from build123d import *

# Parameters (mm, degrees)
SKETCH1_W            = 182
SKETCH1_H            = 33.5
BOSS_EXTRUDE1_DEPTH  = 1.6
SKETCH2_R            = 1.75
CUT_EXTRUDE1_DEPTH   = 1.6
LPATTERN1_COUNT      = 2
LPATTERN1_PITCH      = 175
LPATTERN1_COUNT_DIR2 = 2
LPATTERN1_PITCH_DIR2 = 26.5
SKETCH3_W            = 161.4
SKETCH3_H            = 28.9
BOSS_EXTRUDE2_DEPTH  = 8.95
SKETCH3_2_W          = 161.4
SKETCH3_2_H          = 28.9
BOSS_EXTRUDE3_DEPTH  = 4.65
SKETCH4_W            = 154.4
SKETCH4_H            = 16.5
CUT_EXTRUDE2_DEPTH   = 1
FILLET1_R            = 1
FILLET2_R            = 1
FILLET3_R            = 1
FILLET4_R            = 1


with BuildPart() as part:
    # Sketch1 → Boss-Extrude1 (new body)
    with BuildSketch(Plane(origin=(0, 0, 0), x_dir=(1, 0, 0), z_dir=(0, 1, 0))):
        with Locations((10.727604206, -13.815258398)):
            Rectangle(SKETCH1_W, SKETCH1_H)
    extrude(amount=BOSS_EXTRUDE1_DEPTH)

    # Sketch2 → Cut-Extrude1 (cut)
    with BuildSketch(Plane(origin=(0, 1.6, 0), x_dir=(1, 0, 0), z_dir=(0, 1, 0))):
        with Locations(Location((-76.772395794, -0.565258398, 0), (0, 0, 270))):
            Circle(SKETCH2_R)
    cut_extrude1 = extrude(amount=-CUT_EXTRUDE1_DEPTH, mode=Mode.SUBTRACT)

    # LPattern1: Cut-Extrude1 2 × 2
    with Locations(*[(i * LPATTERN1_PITCH, 0, j * LPATTERN1_PITCH_DIR2) for i in range(LPATTERN1_COUNT) for j in range(LPATTERN1_COUNT_DIR2) if (i, j) != (0, 0)]):
        add(cut_extrude1, mode=Mode.SUBTRACT)

    # Sketch3 → Boss-Extrude2 (add)
    with BuildSketch(Plane(origin=(0, 1.6, 0), x_dir=(1, 0, 0), z_dir=(0, 1, 0))):
        with Locations((13.227604206, -13.815258398)):
            Rectangle(SKETCH3_W, SKETCH3_H)
    extrude(amount=BOSS_EXTRUDE2_DEPTH)

    # Sketch3_2 → Boss-Extrude3 (add)
    with BuildSketch(Plane(origin=(0, 1.6, 0), x_dir=(1, 0, 0), z_dir=(0, 1, 0))):
        with Locations((13.227604206, -13.815258398)):
            Rectangle(SKETCH3_2_W, SKETCH3_2_H)
    extrude(amount=-BOSS_EXTRUDE3_DEPTH)

    # Sketch4 → Cut-Extrude2 (cut)
    with BuildSketch(Plane(origin=(0, 10.55, 0), x_dir=(1, 0, 0), z_dir=(0, 1, 0))):
        with Locations((13.227604206, -13.815258398)):
            Rectangle(SKETCH4_W, SKETCH4_H)
    extrude(amount=-CUT_EXTRUDE2_DEPTH, mode=Mode.SUBTRACT)

    # Fillet1
    fillet1_edges = [part.edges().sort_by_distance(p)[0] for p in [
        (-63.972395794, 10.05, 5.565258398),
    ]]
    fillet(fillet1_edges, radius=FILLET1_R)

    # Fillet2
    fillet2_edges = [part.edges().sort_by_distance(p)[0] for p in [
        (-63.972395794, 10.05, 22.065258398),
    ]]
    fillet(fillet2_edges, radius=FILLET2_R)

    # Fillet3
    fillet3_edges = [part.edges().sort_by_distance(p)[0] for p in [
        (90.427604206, 10.05, 5.565258398),
    ]]
    fillet(fillet3_edges, radius=FILLET3_R)

    # Fillet4
    fillet4_edges = [part.edges().sort_by_distance(p)[0] for p in [
        (90.427604206, 10.05, 22.065258398),
    ]]
    fillet(fillet4_edges, radius=FILLET4_R)


solid = part.part
Could you check a few things on this model? Use its own coordinates, in mm. A direction names the side the tool comes from. Coordinates: 2 decimals unless noted, no trailing zeros. Loops run counter-clockwise (first coordinate to the right, second up) from the corner with the lowest first, then second, coordinate; pieces in that order, holes last.
1. Imagine slicing it at D-D (z = 4). Please give me the cut outline in (x, y).
2. Imagine slicing it at C-C (y = 7). Please give me the cut outline in (x, z).
3. We'd pull the mould along X, two halves only. Please class faces 1 (the face through (93.928, -2, 14)), 2 (the face through (12, 10.55, 4)), 3 (the face through (12, 9.55, 14)): released by +X, released by -X, zero draft, split by the parting line, or undercut.
4. For faces 4 (the face through (12, -2, -0.635)), 5 (the face through (12, 6, 28.265)), 6 (the face through (12, 6, -0.635)), 7 (the face through (12, -2, 28.265)), 8 (the face through (-67.472, 6, 14)), which set-ups out of +Z, -Z, +X, -X, +Y, -Y let a thin tool reach every point of the face, with its end or its side?
5. I need wall thicknesses on L1, parallel to X at y = 1.5, z = -1 (3 decimals); L2, parallel to Z at x = -9.5, y = 9.25; L3, parallel to X at y = 9.25, z = 19.5. Which ranges of each line are inside material? Lowest first, please.
6. Imagine slicing it at B-B (x = -26.5). Please give me the cut outline in (y, z).
7. Imagine slicing it at A-A (z = 18). Please give me the cut outline in (x, y), and give its area (3 significant figures).
8. For P1, Ø8, axis at x = -12.5, z = 13.5, coming from the +Y side; P2, Ø2.5, axis at y = 5.5, z = 10.5, coming from the +X side; P3, Ø3, axis at x = -41.5, y = 7.5, coming from the +Z side; P4, Ø3, axis at x = 98.23, z = 0.57, coming from the +Y side, each with a flat end and sliding along its axis, tell me the tip position at first contact or that it passes through.
Computed values:
1. outline: (-80.27, 0) - (-67.47, 0) - (-67.47, -3.05) - (93.93, -3.05) - (93.93, 0) - (101.73, 0) - (101.73, 1.6) - (93.93, 1.6) - (93.93, 10.55) - (-67.47, 10.55) - (-67.47, 1.6) - (-80.27, 1.6) - close
2. outline: (-67.47, -0.63) - (93.93, -0.63) - (93.93, 28.27) - (-67.47, 28.27) - close
3. face 1: released by +X
3. face 2: zero draft
3. face 3: undercut
4. face 4: -Z, +X, -X, -Y
4. face 5: +Z, +X, -X, +Y
4. face 6: -Z, +X, -X, +Y
4. face 7: +Z, +X, -X, -Y
4. face 8: +Z, -Z, -X, +Y
5. L1: x = -80.272 to -77.555, -75.99 to 97.445, 99.01 to 101.728
5. L2: z = -0.63 to 28.27
5. L3: x = -67.47 to 93.93
6. outline: (-3.05, -0.63) - (0, -0.63) - (0, -2.93) - (1.6, -2.93) - (1.6, -0.63) - (10.55, -0.63) - (10.55, 5.57) - (9.55, 5.57) - (9.55, 22.07) - (10.55, 22.07) - (10.55, 28.27) - (1.6, 28.27) - (1.6, 30.57) - (0, 30.57) - (0, 28.27) - (-3.05, 28.27) - close
7. outline: (-80.27, 0) - (-67.47, 0) - (-67.47, -3.05) - (93.93, -3.05) - (93.93, 0) - (101.73, 0) - (101.73, 1.6) - (93.93, 1.6) - (93.93, 10.55) - (90.43, 10.55) - (90.43, 9.55) - (-63.97, 9.55) - (-63.97, 10.55) - (-67.47, 10.55) - (-67.47, 1.6) - (-80.27, 1.6) - close
7. area: 2,070 mm2
8. P1: stops at y = 9.55
8. P2: stops at x = 93.93
8. P3: stops at z = 28.27
8. P4: passes through
